The model under review builds one solid part; all positions refer to its coordinate system, in mm. Face numbers are marked on the shaded views. A direction names the side the tool comes from. Coordinates: 2 decimals unless noted, no trailing zeros. Write each loop counter-clockwise with the first axis right and the second up, starting at its lowest first coordinate (ties: lowest second). Pieces come first, ordered by that corner, then holes. Notation, with made-up numbers: (-14, 89.5) - (-3, 89.5) arc R27 cw to (-3, 127.5) - close; hole circle Ø5 at (-3.75, 87). An arc over 180 degrees is marked (long way). Put each result on its own line as item: value.
Autodesk Fusion 360 part; units mm, degrees
sketch "Sketch1" plane through (0, 0, 0) normal (0, 0, 1) x (1, 0, 0)
  line L0 (0, 0) -> (50, 0)
  line L1 (50, 0) -> (50, 65)
  line L2 (50, 65) -> (0, 65)
  line L3 (0, 65) -> (0, 0)
  dimension "d1" = 50
  dimension "d2" = 65
extrude "Extrude1" add sketch "Sketch1" along normal blind 3
sketch "Sketch2" plane through (0, 0, 3) normal (0, 0, 1) x (-1, 0, 0)
  line L0 (0, -65) -> (0, 0)
  line L1 (0, 0) -> (-50, 0)
  line L2 (-50, 0) -> (-50, -65)
  line L3 (-50, -65) -> (0, -65)
  line L4 (0, -65) -> (-3, -65)
  line L5 (-3, -65) -> (-3, 0)
  line L6 (-3, 0) -> (0, 0)
  line L7 (0, 0) -> (0, -65)
  dimension "d5" = 65
  dimension "d6" = 50
  dimension "d7" = 3
extrude "Extrude2" add sketch "Sketch2" along normal blind 45 contours L0 L1 L3 L4 L5 L6 L7
sketch "Sketch3" plane through (0, 0, 3) normal (0, 0, 1) x (-1, 0, 0)
  line L0 (-3, -65) -> (-3, 0)
  line L1 (-3, 0) -> (-50, 0)
  line L2 (-50, 0) -> (-50, -65)
  line L3 (-50, -65) -> (-3, -65)
  line L4 (-50, -65) -> (-47, -65)
  line L5 (-47, -65) -> (-47, 0)
  line L6 (-47, 0) -> (-50, 0)
  line L7 (-50, 0) -> (-50, -65)
  dimension "d10" = 3
extrude "Extrude3" add sketch "Sketch3" along normal blind 45 contours L1 L2 L3 L4 L5 L6 L7
sketch "Sketch4" plane through (0, 0, 0) normal (-1, 0, 0) x (0, -1, 0)
  line L0 (-65, 0) -> (0, 0)
  line L1 (0, 0) -> (0, 48)
  line L2 (0, 48) -> (-65, 48)
  line L3 (-65, 48) -> (-65, 0)
  circle A0 centre (-32.5, 20) radius 1
  dimension "d14" = 2
extrude "Extrude4" cut sketch "Sketch4" against normal blind 51 contours A0
sketch "Sketch5" plane through (0, 0, 3) normal (0, 0, 1) x (-1, 0, 0)
  line L0 (-47, 0) -> (-47, -65)
  line L1 (-47, -65) -> (-3, -65)
  line L2 (-3, -65) -> (-3, 0)
  line L3 (-3, 0) -> (-47, 0)
  line L4 (0, 0) -> (-3, 0)
  circle A0 centre (-6, -59) radius 2
  circle A1 centre (-6, -6) radius 2
  circle A2 centre (-44, -6) radius 2
  circle A3 centre (-44, -59) radius 2
  dimension "d21" = 4
  dimension "d22" = 4
  dimension "d25" = 4
  dimension "d28" = 4
extrude "Extrude5" cut sketch "Sketch5" against normal blind 5 contours A0 | A1 | A2 | A3
fillet "Fillet1" radius 1 4 edges at (50, 32.5, 48) (47, 32.5, 48) (3, 32.5, 48) (0, 32.5, 48)
fillet "Fillet2" radius 1 20 edges at (0, 65, 23.5) (0.2929, 65, 47.7071) (1.5, 65, 48) (2.7071, 65, 47.7071) (3, 65, 25) (47, 65, 25) (47.2929, 65, 47.7071) (48.5, 65, 48) (49.7071, 65, 47.7071) (50, 65, 23.5) (0, 0, 23.5) (0.2929, 0, 47.7071) (1.5, 0, 48) (2.7071, 0, 47.7071) (3, 0, 25) (47, 0, 25) (47.2929, 0, 47.7071) (48.5, 0, 48) (49.7071, 0, 47.7071) (50, 0, 23.5)
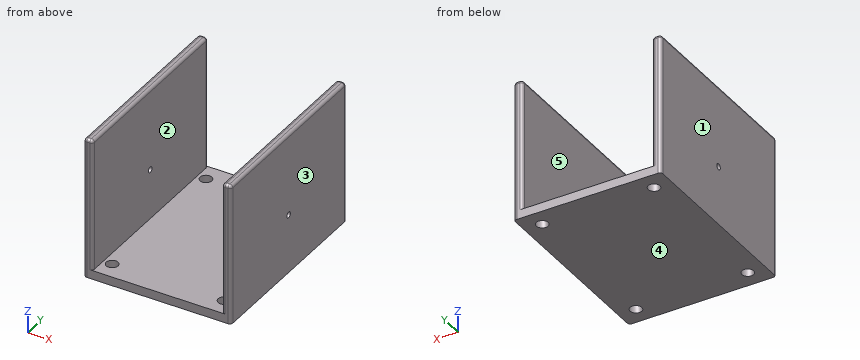
1. For pin 1 Ø8 at (x, y) = (22, 11) entering from -Z; pin 2 Ø1.5 at (x, y) = (27, 15) entering from +Z, all flat-tipped, find the tip position at first contact; note any pin that passes through.
Determined:
pin 1: stops at z = 0
pin 2: stops at z = 3
2. Machinability: for the marked faces 1 and 2, which of the approach directions +Z, -Z, +X, -X, +Y, -Y give a long, thin tool a straight path to every point of the face, cutting with its end or side? Answer none if there is none.
Determined:
face 1: +Z, -Z, -X, +Y, -Y
face 2: +Z, +Y, -Y
3. Consider section B-B on x = 44. State the section outline as (y, z) points.
Determined:
outline: (0, 0) - (4, 0) - (4, 3) - (0, 3) - close; (8, 0) - (57, 0) - (57, 3) - (8, 3) - close; (61, 0) - (65, 0) - (65, 3) - (61, 3) - close
4. Consider section C-C on y = 59. State the section outline as (x, z) points.
Determined:
outline: (0, 0) - (4, 0) - (4, 3) - (3, 3) - (3, 47) arc R1 ccw to (2, 48) - (1, 48) arc R1 ccw to (0, 47) - close; (8, 0) - (42, 0) - (42, 3) - (8, 3) - close; (46, 0) - (50, 0) - (50, 47) arc R1 ccw to (49, 48) - (48, 48) arc R1 ccw to (47, 47) - (47, 3) - (46, 3) - close
5. Consider section A-A on z = 32.5. State the section outline as (x, y) points, plus the area to 3 significant figures.
Determined:
outline: (0, 1) arc R1 ccw to (1, 0) - (2, 0) arc R1 ccw to (3, 1) - (3, 64) arc R1 ccw to (2, 65) - (1, 65) arc R1 ccw to (0, 64) - close; (47, 1) arc R1 ccw to (48, 0) - (49, 0) arc R1 ccw to (50, 1) - (50, 64) arc R1 ccw to (49, 65) - (48, 65) arc R1 ccw to (47, 64) - close
area: 388 mm^2
6. To check wall thickness, follow probe 1 along X at (y, z) = (6, 1); probe 2 along Y at (x, z) = (44, 1); probe 3 along X at (y, z) = (49, 36). State the ranges of each line that lie inside material, in increasing order.
Determined:
probe 1: x = 0 to 4, 8 to 42, 46 to 50
probe 2: y = 0 to 4, 8 to 57, 61 to 65
probe 3: x = 0 to 3, 47 to 50
7. Consider section D-D on z = 20. State the section outline as (x, y) points.
Determined:
outline: (0, 1) arc R1 ccw to (1, 0) - (2, 0) arc R1 ccw to (3, 1) - (3, 31.5) - (0, 31.5) - close; (0, 33.5) - (3, 33.5) - (3, 64) arc R1 ccw to (2, 65) - (1, 65) arc R1 ccw to (0, 64) - close; (47, 1) arc R1 ccw to (48, 0) - (49, 0) arc R1 ccw to (50, 1) - (50, 31.5) - (47, 31.5) - close; (47, 33.5) - (50, 33.5) - (50, 64) arc R1 ccw to (49, 65) - (48, 65) arc R1 ccw to (47, 64) - close
8. The part is to be moulded in two halves that separate along X. For the marked faces 3, 4 and 5, say which applies: +X half, -X half, draft (parallel to the pull), parting line (faces both ways), or undercut.
Determined:
face 3: +X half
face 4: draft
face 5: undercut
